Model file for the job. Use its own axes, mm. Coordinates: 2 decimals unless noted, no trailing zeros. Order: outer loops, then holes, each group sorted by start corner. A loop starts at its lowest first (then second) coordinate and runs counter-clockwise, first axis right, second up.
from build123d import *

# Parameters (mm, degrees)
F0_W     = 255
F0_H     = 250
F0_R     = 6
F0_W_2   = 20
F0_H_2   = 100
F1_DEPTH = 6
F2_W     = 255
F2_H     = 250
F2_W_2   = 20
F2_H_2   = 100
F3_DEPTH = 4


with BuildPart() as f1:
    # F0 (on Top) → F1 (new body)
    with BuildSketch(Plane.XY):
        with Locations((0, -204.858814)):
            Rectangle(F0_W, F0_H)
        with Locations((-112.5, -317.358814)):
            Circle(F0_R, mode=Mode.SUBTRACT)
        with Locations((-87.5, -317.358814)):
            Circle(F0_R, mode=Mode.SUBTRACT)
        with Locations((-112.5, -292.358814)):
            Circle(F0_R, mode=Mode.SUBTRACT)
        with Locations((-87.5, -292.358814)):
            Circle(F0_R, mode=Mode.SUBTRACT)
        with Locations((-62.5, -317.358814)):
            Circle(F0_R, mode=Mode.SUBTRACT)
        with Locations((-37.5, -317.358814)):
            Circle(F0_R, mode=Mode.SUBTRACT)
        with Locations((-12.5, -317.358814)):
            Circle(F0_R, mode=Mode.SUBTRACT)
        with Locations((-62.5, -292.358814)):
            Circle(F0_R, mode=Mode.SUBTRACT)
        with Locations((-37.5, -292.358814)):
            Circle(F0_R, mode=Mode.SUBTRACT)
        with Locations((-12.5, -292.358814)):
            Circle(F0_R, mode=Mode.SUBTRACT)
        with Locations((-112.5, -267.358814)):
            Circle(F0_R, mode=Mode.SUBTRACT)
        with Locations((-87.5, -267.358814)):
            Circle(F0_R, mode=Mode.SUBTRACT)
        with Locations((-87.5, -242.358814)):
            Circle(F0_R, mode=Mode.SUBTRACT)
        with Locations((-107.5, -204.858814)):
            Rectangle(F0_W_2, F0_H_2, mode=Mode.SUBTRACT)
        with Locations((-87.5, -217.358814)):
            Circle(F0_R, mode=Mode.SUBTRACT)
        with Locations((-62.5, -267.358814)):
            Circle(F0_R, mode=Mode.SUBTRACT)
        with Locations((-37.5, -267.358814)):
            Circle(F0_R, mode=Mode.SUBTRACT)
        with Locations((-62.5, -242.358814)):
            Circle(F0_R, mode=Mode.SUBTRACT)
        with Locations((-37.5, -242.358814)):
            Circle(F0_R, mode=Mode.SUBTRACT)
        with Locations((-12.5, -267.358814)):
            Circle(F0_R, mode=Mode.SUBTRACT)
        with Locations((-12.5, -242.358814)):
            Circle(F0_R, mode=Mode.SUBTRACT)
        with Locations((-62.5, -217.358814)):
            Circle(F0_R, mode=Mode.SUBTRACT)
        with Locations((-37.5, -217.358814)):
            Circle(F0_R, mode=Mode.SUBTRACT)
        with Locations((-12.5, -217.358814)):
            Circle(F0_R, mode=Mode.SUBTRACT)
        with Locations((12.5, -317.358814)):
            Circle(F0_R, mode=Mode.SUBTRACT)
        with Locations((37.5, -317.358814)):
            Circle(F0_R, mode=Mode.SUBTRACT)
        with Locations((62.5, -317.358814)):
            Circle(F0_R, mode=Mode.SUBTRACT)
        with Locations((12.5, -292.358814)):
            Circle(F0_R, mode=Mode.SUBTRACT)
        with Locations((37.5, -292.358814)):
            Circle(F0_R, mode=Mode.SUBTRACT)
        with Locations((62.5, -292.358814)):
            Circle(F0_R, mode=Mode.SUBTRACT)
        with Locations((87.5, -317.358814)):
            Circle(F0_R, mode=Mode.SUBTRACT)
        with Locations((112.5, -317.358814)):
            Circle(F0_R, mode=Mode.SUBTRACT)
        with Locations((87.5, -292.358814)):
            Circle(F0_R, mode=Mode.SUBTRACT)
        with Locations((112.5, -292.358814)):
            Circle(F0_R, mode=Mode.SUBTRACT)
        with Locations((12.5, -267.358814)):
            Circle(F0_R, mode=Mode.SUBTRACT)
        with Locations((12.5, -242.358814)):
            Circle(F0_R, mode=Mode.SUBTRACT)
        with Locations((37.5, -267.358814)):
            Circle(F0_R, mode=Mode.SUBTRACT)
        with Locations((62.5, -267.358814)):
            Circle(F0_R, mode=Mode.SUBTRACT)
        with Locations((37.5, -242.358814)):
            Circle(F0_R, mode=Mode.SUBTRACT)
        with Locations((62.5, -242.358814)):
            Circle(F0_R, mode=Mode.SUBTRACT)
        with Locations((12.5, -217.358814)):
            Circle(F0_R, mode=Mode.SUBTRACT)
        with Locations((37.5, -217.358814)):
            Circle(F0_R, mode=Mode.SUBTRACT)
        with Locations((62.5, -217.358814)):
            Circle(F0_R, mode=Mode.SUBTRACT)
        with Locations((87.5, -267.358814)):
            Circle(F0_R, mode=Mode.SUBTRACT)
        with Locations((87.5, -242.358814)):
            Circle(F0_R, mode=Mode.SUBTRACT)
        with Locations((112.5, -267.358814)):
            Circle(F0_R, mode=Mode.SUBTRACT)
        with Locations((87.5, -217.358814)):
            Circle(F0_R, mode=Mode.SUBTRACT)
        with Locations((107.5, -204.858814)):
            Rectangle(F0_W_2, F0_H_2, mode=Mode.SUBTRACT)
        with Locations((-87.5, -192.358814)):
            Circle(F0_R, mode=Mode.SUBTRACT)
        with Locations((-87.5, -167.358814)):
            Circle(F0_R, mode=Mode.SUBTRACT)
        with Locations((-62.5, -192.358814)):
            Circle(F0_R, mode=Mode.SUBTRACT)
        with Locations((-37.5, -192.358814)):
            Circle(F0_R, mode=Mode.SUBTRACT)
        with Locations((-12.5, -192.358814)):
            Circle(F0_R, mode=Mode.SUBTRACT)
        with Locations((-62.5, -167.358814)):
            Circle(F0_R, mode=Mode.SUBTRACT)
        with Locations((-37.5, -167.358814)):
            Circle(F0_R, mode=Mode.SUBTRACT)
        with Locations((-12.5, -167.358814)):
            Circle(F0_R, mode=Mode.SUBTRACT)
        with Locations((-112.5, -142.358814)):
            Circle(F0_R, mode=Mode.SUBTRACT)
        with Locations((-112.5, -117.358814)):
            Circle(F0_R, mode=Mode.SUBTRACT)
        with Locations((-87.5, -142.358814)):
            Circle(F0_R, mode=Mode.SUBTRACT)
        with Locations((-87.5, -117.358814)):
            Circle(F0_R, mode=Mode.SUBTRACT)
        with Locations((-112.5, -92.358814)):
            Circle(F0_R, mode=Mode.SUBTRACT)
        with Locations((-87.5, -92.358814)):
            Circle(F0_R, mode=Mode.SUBTRACT)
        with Locations((-62.5, -142.358814)):
            Circle(F0_R, mode=Mode.SUBTRACT)
        with Locations((-37.5, -142.358814)):
            Circle(F0_R, mode=Mode.SUBTRACT)
        with Locations((-62.5, -117.358814)):
            Circle(F0_R, mode=Mode.SUBTRACT)
        with Locations((-37.5, -117.358814)):
            Circle(F0_R, mode=Mode.SUBTRACT)
        with Locations((-12.5, -142.358814)):
            Circle(F0_R, mode=Mode.SUBTRACT)
        with Locations((-12.5, -117.358814)):
            Circle(F0_R, mode=Mode.SUBTRACT)
        with Locations((-62.5, -92.358814)):
            Circle(F0_R, mode=Mode.SUBTRACT)
        with Locations((-37.5, -92.358814)):
            Circle(F0_R, mode=Mode.SUBTRACT)
        with Locations((-12.5, -92.358814)):
            Circle(F0_R, mode=Mode.SUBTRACT)
        with Locations((12.5, -192.358814)):
            Circle(F0_R, mode=Mode.SUBTRACT)
        with Locations((37.5, -192.358814)):
            Circle(F0_R, mode=Mode.SUBTRACT)
        with Locations((62.5, -192.358814)):
            Circle(F0_R, mode=Mode.SUBTRACT)
        with Locations((12.5, -167.358814)):
            Circle(F0_R, mode=Mode.SUBTRACT)
        with Locations((37.5, -167.358814)):
            Circle(F0_R, mode=Mode.SUBTRACT)
        with Locations((62.5, -167.358814)):
            Circle(F0_R, mode=Mode.SUBTRACT)
        with Locations((87.5, -192.358814)):
            Circle(F0_R, mode=Mode.SUBTRACT)
        with Locations((87.5, -167.358814)):
            Circle(F0_R, mode=Mode.SUBTRACT)
        with Locations((12.5, -142.358814)):
            Circle(F0_R, mode=Mode.SUBTRACT)
        with Locations((12.5, -117.358814)):
            Circle(F0_R, mode=Mode.SUBTRACT)
        with Locations((37.5, -142.358814)):
            Circle(F0_R, mode=Mode.SUBTRACT)
        with Locations((62.5, -142.358814)):
            Circle(F0_R, mode=Mode.SUBTRACT)
        with Locations((37.5, -117.358814)):
            Circle(F0_R, mode=Mode.SUBTRACT)
        with Locations((62.5, -117.358814)):
            Circle(F0_R, mode=Mode.SUBTRACT)
        with Locations((12.5, -92.358814)):
            Circle(F0_R, mode=Mode.SUBTRACT)
        with Locations((37.5, -92.358814)):
            Circle(F0_R, mode=Mode.SUBTRACT)
        with Locations((62.5, -92.358814)):
            Circle(F0_R, mode=Mode.SUBTRACT)
        with Locations((87.5, -142.358814)):
            Circle(F0_R, mode=Mode.SUBTRACT)
        with Locations((87.5, -117.358814)):
            Circle(F0_R, mode=Mode.SUBTRACT)
        with Locations((112.5, -142.358814)):
            Circle(F0_R, mode=Mode.SUBTRACT)
        with Locations((112.5, -117.358814)):
            Circle(F0_R, mode=Mode.SUBTRACT)
        with Locations((87.5, -92.358814)):
            Circle(F0_R, mode=Mode.SUBTRACT)
        with Locations((112.5, -92.358814)):
            Circle(F0_R, mode=Mode.SUBTRACT)
    extrude(amount=F1_DEPTH)

    # F2 (on face) → F3 (join)
    with BuildSketch(Plane(origin=(0, 0, 0), x_dir=(1, 0, 0), z_dir=(0, 0, -1))):
        with Locations((0, 204.858814)):
            Rectangle(F2_W, F2_H)
        with Locations((-107.5, 204.858814)):
            Rectangle(F2_W_2, F2_H_2, mode=Mode.SUBTRACT)
        with Locations((107.5, 204.858814)):
            Rectangle(F2_W_2, F2_H_2, mode=Mode.SUBTRACT)
    extrude(amount=F3_DEPTH)


solid = f1.part
Q1. Mould opens along Y. For faces 1 (the face through (-68.494, -192.095, 2.958)), 2 (the face through (-2, -79.859, 1)) say: pulls with the +Y half, pulls with the -Y half, needs draft (parallel to the pull), parting line crosses it, or undercut.
Established:
face 1: undercut
face 2: pulls with the +Y half
Q2. Cut at A-A, the plane y = -181. List the corners of the cut face in (x, z).
Established:
outline: (-127.5, -4) - (-117.5, -4) - (-117.5, 6) - (-127.5, 6) - close; (-97.5, -4) - (97.5, -4) - (97.5, 6) - (-97.5, 6) - close; (117.5, -4) - (127.5, -4) - (127.5, 6) - (117.5, 6) - close
Q3. Drop flat-ended pins along their axis: P1, Ø7, axis at x = -62.5, y = -142.36, coming from the +Z side; P2, Ø14, axis at x = 12.5, y = -92.36, coming from the +Z side. Give the stop position or say it passes through.
Established:
P1: stops at z = 0
P2: stops at z = 6
Q4. Cut at C-C, the plane z = 3.5. Count the separate pieces of the cut face and the enclosed holes in it, plus the area to 3 significant figures.
Established:
separate pieces: 1
enclosed holes: 94
area: 49,300 mm2
Q5. Probe line 1 (X direction, y = -166, z = -2.5); line 2 (Y direction, x = -98.5, z = 5.75); line 3 (Z direction, x = -86.5, y = -261.5). List the from-to ranges inside material, lowest first.
Established:
line 1: x = -127.5 to -117.5, -97.5 to 97.5, 117.5 to 127.5
line 2: y = -329.86 to -254.86, -154.86 to -79.86
line 3: z = -4 to 0
